from build123d import *

# Parameters (mm, degrees)
SKETCH1_R           = 2.75
SKETCH1_R_2         = 1.5
BOSS_EXTRUDE1_DEPTH = 2.5
FILLET1_R           = 2
BOSS_EXTRUDE2_START = 21.5
BOSS_EXTRUDE2_DEPTH = 21.5
CUT_EXTRUDE1_DEPTH  = 0.5
BOSS_EXTRUDE3_DEPTH = 10


with BuildPart() as part:
    # Sketch1 → Boss-Extrude1 (new body)
    # profile 1 of 3: a face of its own
    with BuildSketch(Plane(origin=(0, 0, 0), x_dir=(1, 0, 0), z_dir=(0, 1, 0))):
        with BuildLine():
            Line((11.139087297, 9.5), (-11.139087297, 9.5))
            Line((-11.139087297, 9.5), (-18.694543648, 1.944543648))
            ThreePointArc((-18.694543648, 1.944543648), (-15.697620561, 2.540668714), (-14, 0))
            ThreePointArc((-14, 0), (-15.697620561, -2.540668714), (-18.694543648, -1.944543648))
            Line((-18.694543648, -1.944543648), (-11.139087297, -9.5))
            Line((-11.139087297, -9.5), (11.139087297, -9.5))
            Line((11.139087297, -9.5), (18.694543648, -1.944543648))
            ThreePointArc((18.694543648, -1.944543648), (14, 0), (18.694543648, 1.944543648))
            Line((18.694543648, 1.944543648), (11.139087297, 9.5))
        make_face()
    # profile 2 of 3: a face of its own
    with BuildSketch(Plane(origin=(0, 0, 0), x_dir=(1, 0, 0), z_dir=(0, 1, 0))):
        with Locations((-16.75, 0)):
            Circle(SKETCH1_R)
        with Locations(Location((-16.75, 0, 0), (0, 0, 270))):
            Circle(SKETCH1_R_2, mode=Mode.SUBTRACT)
    # profile 3 of 3: a face of its own
    with BuildSketch(Plane(origin=(0, 0, 0), x_dir=(1, 0, 0), z_dir=(0, 1, 0))):
        with Locations((16.75, 0)):
            Circle(SKETCH1_R)
        with Locations(Location((16.75, 0, 0), (0, 0, 270))):
            Circle(SKETCH1_R_2, mode=Mode.SUBTRACT)
    extrude(amount=BOSS_EXTRUDE1_DEPTH)

    # Fillet1
    fillet1_edges = [part.edges().sort_by_distance(p)[0] for p in [
        (11.139087297, 1.25, 9.5),
        (-11.139087297, 1.25, 9.5),
        (-11.139087297, 1.25, -9.5),
        (11.139087297, 1.25, -9.5),
    ]]
    fillet(fillet1_edges, radius=FILLET1_R)

    # Sketch3 → Boss-Extrude2 (add)
    with BuildSketch(Plane(origin=(0, 2.5, 0), x_dir=(1, 0, 0), z_dir=(0, 1, 0)).offset(BOSS_EXTRUDE2_START)):
        with BuildLine():
            Line((10.310660172, 9.5), (-10.310660172, 9.5))
            ThreePointArc((-10.310660172, 9.5), (-11.076027037, 9.347759065), (-11.724873734, 8.914213562))
            Line((-11.724873734, 8.914213562), (-11.724873734, -8.914213562))
            ThreePointArc((-11.724873734, -8.914213562), (-11.076027037, -9.347759065), (-10.310660172, -9.5))
            Line((-10.310660172, -9.5), (10.310660172, -9.5))
            ThreePointArc((10.310660172, -9.5), (11.076027037, -9.347759065), (11.724873734, -8.914213562))
            Line((11.724873734, -8.914213562), (11.724873734, 8.914213562))
            ThreePointArc((11.724873734, 8.914213562), (11.076027037, 9.347759065), (10.310660172, 9.5))
        make_face()
    extrude(amount=-BOSS_EXTRUDE2_DEPTH)

    # Sketch4 → Cut-Extrude1 (cut)
    with BuildSketch(Plane(origin=(0, 24, 0), x_dir=(1, 0, 0), z_dir=(0, 1, 0))):
        with BuildLine():
            Line((10.724873734, -8.410179721), (10.724873734, 8.410179721))
            ThreePointArc((10.724873734, 8.410179721), (10.522580297, 8.47728699), (10.310660172, 8.5))
            Line((10.310660172, 8.5), (-10.310660172, 8.5))
            ThreePointArc((-10.310660172, 8.5), (-10.522580297, 8.47728699), (-10.724873734, 8.410179721))
            Line((-10.724873734, 8.410179721), (-10.724873734, -8.410179721))
            ThreePointArc((-10.724873734, -8.410179721), (-10.522580297, -8.47728699), (-10.310660172, -8.5))
            Line((-10.310660172, -8.5), (10.310660172, -8.5))
            ThreePointArc((10.310660172, -8.5), (10.522580297, -8.47728699), (10.724873734, -8.410179721))
        make_face()
    extrude(amount=-CUT_EXTRUDE1_DEPTH, mode=Mode.SUBTRACT)

    # Sketch5 → Boss-Extrude3 (add)
    with BuildSketch(Plane(origin=(0, 23.5, 0), x_dir=(1, 0, 0), z_dir=(0, 1, 0))):
        with BuildLine():
            Line((-8.25, 1), (-8.25, -1))
            ThreePointArc((-8.25, -1), (-9, -1.75), (-9.75, -1))
            Line((-9.75, -1), (-9.75, 1))
            ThreePointArc((-9.75, 1), (-9, 1.75), (-8.25, 1))
        make_face()
        with BuildLine():
            Line((8.25, 1), (8.25, -1))
            ThreePointArc((8.25, -1), (9, -1.75), (9.75, -1))
            Line((9.75, -1), (9.75, 1))
            ThreePointArc((9.75, 1), (9, 1.75), (8.25, 1))
        make_face()
    extrude(amount=BOSS_EXTRUDE3_DEPTH)


solid = part.part
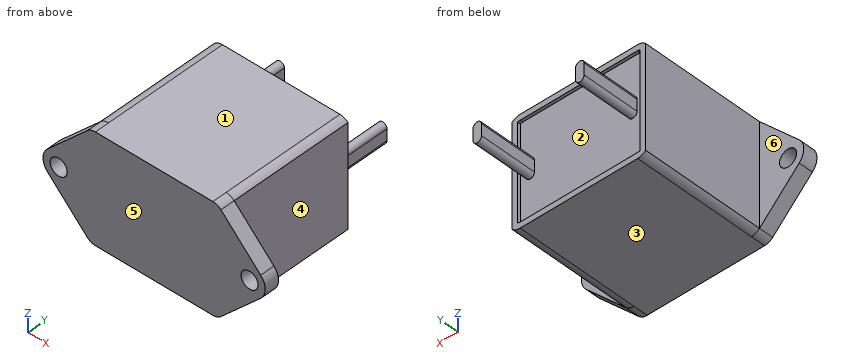
The listing builds one solid part. Answer for the finished solid, in the listing's coordinates (mm). Face numbers are marked on the shaded views. A direction names the side the tool comes from. Round coordinates to 2 decimals unless told otherwise and drop trailing zeros. Loops run counter-clockwise (first coordinate to the right, second up) from the corner with the lowest first, then second, coordinate; pieces in that order, holes last. Notation, with made-up numbers: M 57,42.5 L 112,42.5 A23 ccw 112,77.5 Z; hole C 84,56 d8. An arc over 180 degrees is marked long. Write each question's results on one line, items separated by ' | '. Start each with the question number.
1) Find section D-D on z = -3.5. Write down the section's boundary in (x, y), plus the area to 3 significant figures.
2) Find section C-C on y = 15. Write down the section's boundary in (x, z).
3) Determine the mould class of the marked faces 1, 2, 3 and 4 for opening direction Z: pulls with the +Z half, pulls with the -Z half, needs draft (parallel to the pull), parting line crosses it, or undercut.
4) Find section A-A on y = 26. Write down the section's boundary in (x, z), plus the area to 3 significant figures.
5) Find section B-B on x = 1. Write down the section's boundary in (y, z).
6) Each of these flat-tipped pins is pushed along its axis until it touches: pin 1 (8.5 mm diameter, centred on x = 16.5, z = -2.5, fed in from +Y); pin 2 (8 mm diameter, centred on y = 18.5, z = -3.5, fed in from -X); pin 3 (2 mm diameter, centred on y = 27, z = 0, fed in from -X); pin 4 (4 mm diameter, centred on x = -12.5, y = 26, fed in from -Z). Where does it stop, or does it pass through?
7) Which of the six approach directions +Z, -Z, +X, -X, +Y, -Y give full straight-line access (tool end or side, diameter ignored) to the marked faces 5 and 6?
8) Straight lines are drawn through the part: probe 1 along X at (y, z) = (1, 0); probe 2 along X at (y, z) = (30, -0.5); probe 3 along Y at (x, z) = (14, -3). For each, find the intervals that lie inside material, in ascending order.
Final values:
1) outline: M -17.14,0 L 17.14,0 L 17.14,2.5 L 11.72,2.5 L 11.72,24 L 10.72,24 L 10.72,23.5 L -10.72,23.5 L -10.72,24 L -11.72,24 L -11.72,2.5 L -17.14,2.5 Z | area: 579 mm²
2) outline: M -11.72,-8.91 A2 ccw -10.31,-9.5 L 10.31,-9.5 A2 ccw 11.72,-8.91 L 11.72,8.91 A2 ccw 10.31,9.5 L -10.31,9.5 A2 ccw -11.72,8.91 Z
3) face 1: pulls with the +Z half | face 2: undercut | face 3: pulls with the -Z half | face 4: needs draft
4) outline: M -9.75,-1 A0.75 ccw -8.25,-1 L -8.25,1 A0.75 ccw -9.75,1 Z; M 8.25,-1 A0.75 ccw 9.75,-1 L 9.75,1 A0.75 ccw 8.25,1 Z | area: 9.53 mm²
5) outline: M 0,-9.5 L 24,-9.5 L 24,-8.5 L 23.5,-8.5 L 23.5,8.5 L 24,8.5 L 24,9.5 L 0,9.5 Z
6) pin 1: y = 2.5 | pin 2: x = -11.72 | pin 3: x = -9.75 | pin 4: through
7) face 5: +Z, -Z, +X, -X, -Y | face 6: +Z, -Z, -X, +Y
8) probe 1: -19.5 to -18.25, -15.25 to 15.25, 18.25 to 19.5 | probe 2: -9.75 to -8.25, 8.25 to 9.75 | probe 3: 0 to 2.5
